```python
from build123d import *
from build123d.topology import SkipClean

# Parameters (mm, degrees)
SKETCH1_W                = 100
SKETCH1_H                = 80
SKETCH1_R                = 10
SKETCH1_R_2              = 1.65
BOSS_EXTRUDE1_DEPTH      = 6.35
SKETCH3_R                = 2
CUT_EXTRUDE5_DEPTH       = 65.345337826
BOSS_EXTRUDE2_DEPTH      = 6.35
SKETCH6_W                = 105.351133128
SKETCH6_H                = 40
CUT_EXTRUDE6_DEPTH       = 69.586226304
SKETCH7_R                = 3.5
CUT_EXTRUDE7_DEPTH       = 3
BOSS_EXTRUDE4_START      = -6.35
BOSS_EXTRUDE4_DEPTH      = 46.35
SKETCH9_R                = 3.497663505
CUT_EXTRUDE8_DEPTH       = 25
CUT_EXTRUDE9_START       = 25
SKETCH10_R               = 3.529979832
SKETCH10_R_2             = 2
CUT_EXTRUDE9_DEPTH       = 25
SKETCH12_R               = 2.238504643
CUT_EXTRUDE10_DEPTH      = 25
SKETCH13_R               = 7.75
CUT_EXTRUDE11_DEPTH      = 25
SKETCH14_R               = 1.7
CUT_EXTRUDE12_DEPTH      = 10
SKETCH16_W               = 1.6
SKETCH16_H               = 11.621506057
BOSS_EXTRUDE5_DEPTH      = 8
CHAMFER1_SIZE            = 5
CHAMFER2_SIZE            = 5
CUT_EXTRUDE13_DEPTH      = 8
CUT_EXTRUDE13_DEPTH_BACK = 1.6
SKETCH17_R               = 2
SKETCH18_W               = 5
SKETCH18_H               = 11.621506057
BOSS_EXTRUDE6_DEPTH      = 2


with BuildPart() as part:
    # Sketch1 → Boss-Extrude1 (new body)
    with BuildSketch(Plane(origin=(0, 0, 0), x_dir=(1, 0, 0), z_dir=(0, 1, 0))):
        Rectangle(SKETCH1_W, SKETCH1_H)
        with Locations(Location((0, -20, 0), (0, 0, 270))):
            Circle(SKETCH1_R, mode=Mode.SUBTRACT)
        with Locations(Location((23, -29, 0), (0, 0, 270))):
            Circle(SKETCH1_R_2, mode=Mode.SUBTRACT)
        with Locations(Location((47, -11, 0), (0, 0, 270))):
            Circle(SKETCH1_R_2, mode=Mode.SUBTRACT)
        with Locations(Location((23, -11, 0), (0, 0, 270))):
            Circle(SKETCH1_R_2, mode=Mode.SUBTRACT)
        with Locations(Location((47, -29, 0), (0, 0, 270))):
            Circle(SKETCH1_R_2, mode=Mode.SUBTRACT)
        with Locations(Location((-23, -29, 0), (0, 0, 90))):
            Circle(SKETCH1_R_2, mode=Mode.SUBTRACT)
        with Locations(Location((-47, -29, 0), (0, 0, 90))):
            Circle(SKETCH1_R_2, mode=Mode.SUBTRACT)
        with Locations(Location((-47, -11, 0), (0, 0, 90))):
            Circle(SKETCH1_R_2, mode=Mode.SUBTRACT)
        with Locations(Location((-23, -11, 0), (0, 0, 90))):
            Circle(SKETCH1_R_2, mode=Mode.SUBTRACT)
    extrude(amount=BOSS_EXTRUDE1_DEPTH)

    # Sketch3 → Cut-Extrude5 (cut, through all)
    with BuildSketch(Plane(origin=(0, 6.35, 0), x_dir=(1, 0, 0), z_dir=(0, 1, 0))):
        with Locations((50, -20)):
            Circle(SKETCH3_R)
        with Locations(Location((-10, -35, 0), (0, 0, 270))):
            Circle(SKETCH3_R)
        with Locations(Location((-10, -5, 0), (0, 0, 90))):
            Circle(SKETCH3_R)
    extrude(amount=-CUT_EXTRUDE5_DEPTH, mode=Mode.SUBTRACT)

    # Sketch5 → Boss-Extrude2 (add)
    with SkipClean():  # the faces are left unmerged after this step: merging them gives an invalid solid
        with BuildSketch(Plane(origin=(0, 6.35, 0), x_dir=(1, 0, 0), z_dir=(0, 1, 0))):
            with BuildLine():
                Line((50, -22), (50, -40))
                Line((50, -40), (55.351133128, -40))
                Line((55.351133128, -40), (55.351133128, 40))
                Line((55.351133128, 40), (50, 40))
                Line((50, 40), (50, -18))
                ThreePointArc((50, -18), (52, -20), (50, -22))
            make_face()
        extrude(amount=-BOSS_EXTRUDE2_DEPTH)

    # Sketch6 → Cut-Extrude6 (cut, through all)
    with SkipClean():  # the faces are left unmerged after this step: merging them gives an invalid solid
        with BuildSketch(Plane(origin=(0, 6.35, 0), x_dir=(1, 0, 0), z_dir=(0, 1, 0))):
            with Locations((2.675566564, 20)):
                Rectangle(SKETCH6_W, SKETCH6_H)
        extrude(amount=-CUT_EXTRUDE6_DEPTH, mode=Mode.SUBTRACT)

    # Sketch7 → Cut-Extrude7 (cut)
    with SkipClean():  # the faces are left unmerged after this step: merging them gives an invalid solid
        with BuildSketch(Plane(origin=(0, 6.35, 0), x_dir=(1, 0, 0), z_dir=(0, 1, 0))):
            with Locations(Location((-10, -5, 0), (0, 0, 270))):
                Circle(SKETCH7_R)
            with Locations(Location((-10, -35, 0), (0, 0, 270))):
                Circle(SKETCH7_R)
            with Locations(Location((50, -20, 0), (0, 0, 270))):
                Circle(SKETCH7_R)
        extrude(amount=-CUT_EXTRUDE7_DEPTH, mode=Mode.SUBTRACT)

    # Sketch8 → Boss-Extrude4 (add)
    with BuildSketch(Plane(origin=(0, 6.35, 0), x_dir=(1, 0, 0), z_dir=(0, 1, 0)).offset(BOSS_EXTRUDE4_START)):
        with BuildLine():
            Line((-47, -9.35), (-23, -9.35))
            ThreePointArc((-23, -9.35), (-21.833273811, -9.833273811), (-21.35, -11))
            Line((-21.35, -11), (-21.35, -29))
            ThreePointArc((-21.35, -29), (-21.833273811, -30.166726189), (-23, -30.65))
            Line((-23, -30.65), (-47, -30.65))
            ThreePointArc((-47, -30.65), (-48.166726189, -30.166726189), (-48.65, -29))
            Line((-48.65, -29), (-48.65, -11))
            ThreePointArc((-48.65, -11), (-48.166726189, -9.833273811), (-47, -9.35))
        make_face()
        with BuildLine():
            Line((21.35, -11), (21.35, -29))
            ThreePointArc((21.35, -29), (21.833273811, -30.166726189), (23, -30.65))
            Line((23, -30.65), (47, -30.65))
            ThreePointArc((47, -30.65), (48.166726189, -30.166726189), (48.65, -29))
            Line((48.65, -29), (48.65, -11))
            ThreePointArc((48.65, -11), (48.166726189, -9.833273811), (47, -9.35))
            Line((47, -9.35), (23, -9.35))
            ThreePointArc((23, -9.35), (21.833273811, -9.833273811), (21.35, -11))
        make_face()
    extrude(amount=BOSS_EXTRUDE4_DEPTH)

    # Sketch9 → Cut-Extrude8 (cut)
    with BuildSketch(Plane(origin=(0, 6.35, 0), x_dir=(1, 0, 0), z_dir=(0, 1, 0))):
        with Locations((50, -20)):
            Circle(SKETCH9_R)
    extrude(amount=CUT_EXTRUDE8_DEPTH, mode=Mode.SUBTRACT)

    # Sketch10 → Cut-Extrude9 (cut)
    with BuildSketch(Plane(origin=(0, 3.35, 0), x_dir=(1, 0, 0), z_dir=(0, 1, 0)).offset(CUT_EXTRUDE9_START)):
        with Locations(Location((50, -20, 0), (0, 0, 112.484807611))):
            Circle(SKETCH10_R)
        with Locations((50, -20)):
            Circle(SKETCH10_R_2, mode=Mode.SUBTRACT)
    extrude(amount=-CUT_EXTRUDE9_DEPTH, mode=Mode.SUBTRACT)

    # Sketch12 → Cut-Extrude10 (cut)
    with BuildSketch(Plane.XZ):
        with Locations(Location((50, 20, 0), (0, 0, 270))):
            Circle(SKETCH12_R)
    extrude(amount=-CUT_EXTRUDE10_DEPTH, mode=Mode.SUBTRACT)

    # Sketch13 → Cut-Extrude11 (cut)
    with BuildSketch(Plane.XY.offset(30.65)):
        with Locations((35, 34.35)):
            Circle(SKETCH13_R)
        with Locations(Location((-35, 34.35, 0), (0, 0, 180))):
            Circle(SKETCH13_R)
    extrude(amount=-CUT_EXTRUDE11_DEPTH, mode=Mode.SUBTRACT)

    # Sketch14 → Cut-Extrude12 (cut)
    with BuildSketch(Plane(origin=(0, 46.35, 0), x_dir=(1, 0, 0), z_dir=(0, 1, 0))):
        with Locations(Location((35, -20, 0), (0, 0, 270))):
            Circle(SKETCH14_R)
        with Locations(Location((-35, -20, 0), (0, 0, 270))):
            Circle(SKETCH14_R)
    extrude(amount=-CUT_EXTRUDE12_DEPTH, mode=Mode.SUBTRACT)

    # Sketch16 → Boss-Extrude5 (add)
    with BuildSketch(Plane(origin=(0, 6.35, 0), x_dir=(1, 0, 0), z_dir=(0, 1, 0))):
        with Locations((10.7, -34.189246971)):
            Rectangle(SKETCH16_W, SKETCH16_H)
        with Locations((7.3, -5.810753029)):
            Rectangle(SKETCH16_W, SKETCH16_H)
        with Locations((10.7, -5.810753029)):
            Rectangle(SKETCH16_W, SKETCH16_H)
        with Locations((7.3, -34.189246971)):
            Rectangle(SKETCH16_W, SKETCH16_H)
    extrude(amount=BOSS_EXTRUDE5_DEPTH)

    # Chamfer1
    chamfer1_edges = [part.edges().sort_by_distance(p)[0] for p in [
        (11.5, 6.35, 5.810753029),
        (11.5, 6.35, 34.189246971),
    ]]
    chamfer(chamfer1_edges, length=CHAMFER1_SIZE)

    # Chamfer2
    # the kernel refuses this chamfer: 5 mm, written as the material it adds along each edge
    with BuildSketch(Plane(origin=(6.5, 6.35, 0), x_dir=(0.027495876610586317, 0.9996219169112968, 0), z_dir=(0, 0, 1))) as chamfer2_piece_1_section:
        Polygon((CHAMFER2_SIZE * 0.999621916911, CHAMFER2_SIZE * 0.0274958766106), (-CHAMFER2_SIZE * 0.0274958766106, CHAMFER2_SIZE * 0.999621916911), (0, 0), align=None)
    chamfer2_piece_1 = extrude(amount=11.621506057, mode=Mode.PRIVATE)
    chamfer2_piece_1 = chamfer2_piece_1 - Plane(origin=(0, 8.026002071, 20), x_dir=(0, 0, 1), z_dir=(0, -1, 0)) * Cylinder(10, 44, mode=Mode.PRIVATE)
    add(chamfer2_piece_1)
    with BuildSketch(Plane(origin=(6.5, 6.35, 28.378493943), x_dir=(0.027495876610586317, 0.9996219169112968, 0), z_dir=(0, 0, 1))) as chamfer2_piece_2_section:
        Polygon((CHAMFER2_SIZE * 0.999621916911, CHAMFER2_SIZE * 0.0274958766106), (-CHAMFER2_SIZE * 0.0274958766106, CHAMFER2_SIZE * 0.999621916911), (0, 0), align=None)
    chamfer2_piece_2 = extrude(amount=11.621506057, mode=Mode.PRIVATE)
    chamfer2_piece_2 = chamfer2_piece_2 - Plane(origin=(0, 8.026002093, 20), x_dir=(0, 0, 1), z_dir=(0, -1, 0)) * Cylinder(10, 44, mode=Mode.PRIVATE)
    add(chamfer2_piece_2)

    # Sketch17 → Cut-Extrude13 (cut, two sides: drawn at the far end of the back side and taken through both)
    with BuildSketch(Plane(origin=(11.5, 0, 0), x_dir=(0, 0, -1), z_dir=(1, 0, 0)).offset(-CUT_EXTRUDE13_DEPTH_BACK)):
        with Locations(Location((-5.810753029, 10.35, 0), (0, 0, 150))):
            Circle(SKETCH17_R)
        with Locations(Location((-34.189246971, 10.35, 0), (0, 0, 150))):
            Circle(SKETCH17_R)
    extrude(amount=CUT_EXTRUDE13_DEPTH + CUT_EXTRUDE13_DEPTH_BACK, mode=Mode.SUBTRACT)

    # Sketch18 → Boss-Extrude6 (add)
    with BuildSketch(Plane(origin=(0, 14.35, 0), x_dir=(1, 0, 0), z_dir=(0, 1, 0))):
        with Locations((9, -5.810753029)):
            Rectangle(SKETCH18_W, SKETCH18_H)
        with Locations((9, -34.189246971)):
            Rectangle(SKETCH18_W, SKETCH18_H)
    extrude(amount=BOSS_EXTRUDE6_DEPTH)


solid = part.part
```
The listing builds one solid part. Answer for the finished solid, in the listing's coordinates (mm). A direction names the side the tool comes from. Coordinates: 2 decimals unless noted, no trailing zeros. Order: outer loops, then holes, each group sorted by start corner. A loop starts at its lowest first (then second) coordinate and runs counter-clockwise, first axis right, second up. Notation, with made-up numbers: M 1,50.5 L 45,50.5 A31 ccw 45,87.5 Z; hole C 82.5,-37.5 d7. An arc over 180 degrees is marked long. Answer as a JSON object with one key per item and string values. Group by question number.
1. A tool of negligible diameter and unlimited length cuts with its end or side. For faces 5 (the flat face through (48.65, 26, 16)), 6 (the cylindrical face through (-9.846, 4.871, 31.503)), 7 (the flat face through (-48.65, 26, 20)), from which of +Z, -Z, +X, -X, +Y, -Y can it reach the whole face along a straight path? Write none if from no direction.
2. Section A-A on y = 34.35 is taken. Write down the section's boundary in (x, z).
3. Section B-B on x = 35 is taken. Write down the section's boundary in (y, z), then the cut area to 3 significant figures.
4. Straight lines are drawn through the part: line 1 (X direction, y = 44.3, z = 20); line 2 (X direction, y = 12.5, z = 24.5); line 3 (Z direction, x = 0, y = 2.5). For each, find the intervals that lie inside material, in ascending order.
5. Section D-D on y = 19.5 is taken. Write down the section's boundary in (x, z).
6. Determine the mould class of faces 1 (the flat face through (55.351, 3, 20)), 2 (the flat face through (49.3, 3.35, 22.3)), 3 (the cylindrical face through (46.524, 13.247, 19.385)), 4 (the flat face through (-35, 46.35, 22)) for opening direction X: released by +X, released by -X, zero draft, split by the parting line, or undercut.
7. Flat-ended cylindrical pins translate along their axes: P1, Ø5, axis at x = 10, z = 19.5, coming from the +Y side; P2, Ø10, axis at y = 15, z = 10, coming from the -X side; P3, Ø6.5, axis at y = 11, z = 5.5, coming from the +X side. Find the tip coordinate at first contact, or state that the pin passes through.
8. Section C-C on z = 20 is taken. State how many separate pieces and enclosed holes the cut face has, then the cut area to 3 significant figures.
Values follow:
{
 "1": {"face 5": "+Z, -Z, +X, +Y", "face 6": "+Y", "face 7": "+Z, -Z, -X, +Y"},
 "2": {"outline": "M -48.65,11 A1.65 ccw -47,9.35 L -42.75,9.35 L -42.75,30.65 L -47,30.65 A1.65 ccw -48.65,29 Z; M -27.25,9.35 L -23,9.35 A1.65 ccw -21.35,11 L -21.35,29 A1.65 ccw -23,30.65 L -27.25,30.65 Z; M 21.35,11 A1.65 ccw 23,9.35 L 27.25,9.35 L 27.25,30.65 L 23,30.65 A1.65 ccw 21.35,29 Z; M 42.75,9.35 L 47,9.35 A1.65 ccw 48.65,11 L 48.65,29 A1.65 ccw 47,30.65 L 42.75,30.65 Z"},
 "3": {"outline": "M 0,0 L 6.35,0 L 6.35,9.35 L 26.6,9.35 L 26.6,30.65 L 6.35,30.65 L 6.35,40 L 0,40 Z; M 42.1,9.35 L 46.35,9.35 L 46.35,18.3 L 42.1,18.3 Z; M 42.1,21.7 L 46.35,21.7 L 46.35,30.65 L 42.1,30.65 Z", "area": "761 mm2"},
 "4": {"line 1": "-48.65 to -36.7, -33.3 to -21.35, 21.35 to 33.3, 36.7 to 48.65", "line 2": "-48.65 to -21.35, 21.35 to 48.65", "line 3": "0 to 10, 30 to 40"},
 "5": {"outline": "M -48.65,11 A1.65 ccw -47,9.35 L -23,9.35 A1.65 ccw -21.35,11 L -21.35,29 A1.65 ccw -23,30.65 L -47,30.65 A1.65 ccw -48.65,29 Z; M 21.35,11 A1.65 ccw 23,9.35 L 47,9.35 A1.65 ccw 48.65,11 L 48.65,16.74 A3.53 cw 48.65,23.26 L 48.65,29 A1.65 ccw 47,30.65 L 23,30.65 A1.65 ccw 21.35,29 Z"},
 "6": {"face 1": "released by +X", "face 2": "undercut", "face 3": "undercut", "face 4": "zero draft"},
 "7": {"P1": "y = 6.35", "P2": "x = -48.65", "P3": "x = 15.1"},
 "8": {"separate pieces": "3", "enclosed holes": "0", "area": "2,230 mm2"}
}
